Answer from the drawing. Dimensions are ordinates in mm from the lowest x, y and z of the part. A direction names the side the tool comes from. Round coordinates to 2 decimals unless told otherwise and drop trailing zeros. Loops run counter-clockwise (first coordinate to the right, second up) from the corner with the lowest first, then second, coordinate; pieces in that order, holes last. Notation, with made-up numbers: M -6.75,58.25 L 46.25,58.25 A25 cw 46.25,93.25 Z; hole C -38,-9 d8. An arc over 180 degrees is marked long. Answer as a JSON object with one key per item and string values.
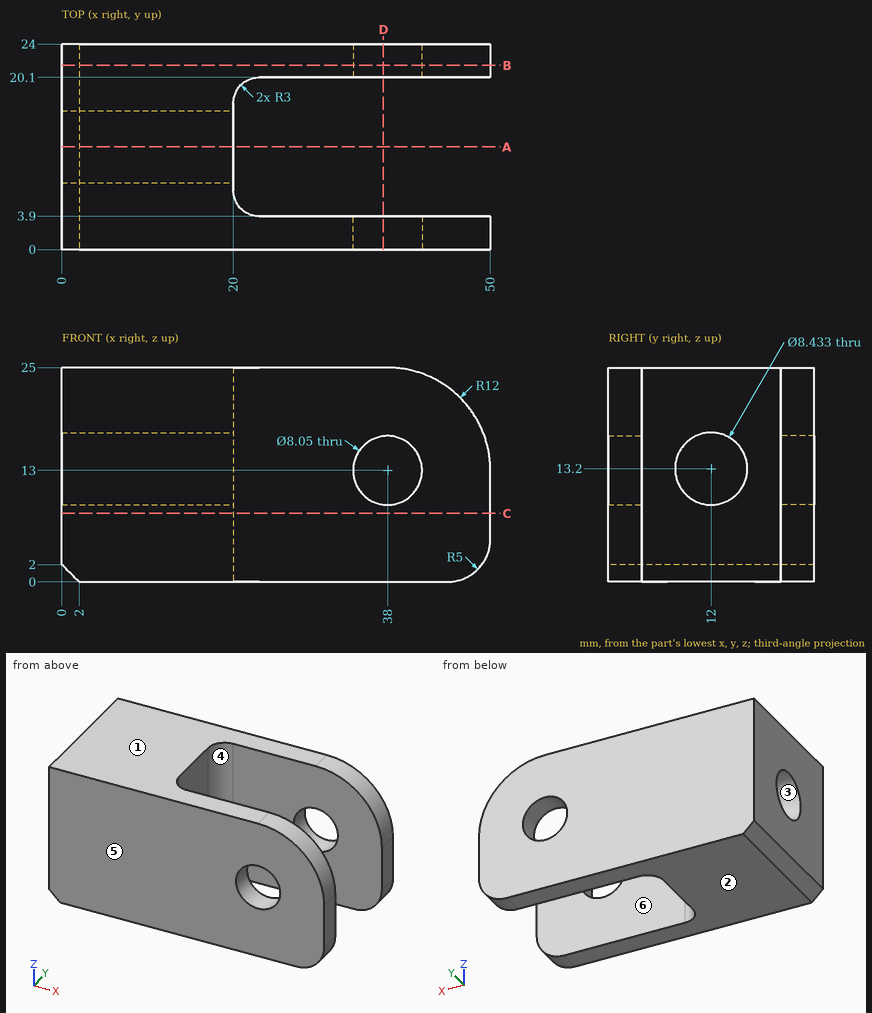
Item 1: Which of the six approach directions +Z, -Z, +X, -X, +Y, -Y give full straight-line access (tool end or side, diameter ignored) to the marked faces 5 and 6?
Values follow:
{"face 5": "+Z, -Z, +X, -X, -Y", "face 6": "+Z, -Z, +X"}
Item 2: Determine the mould class of the marked faces 1, 2, 3 and 4 for opening direction Z: released by +Z, released by -Z, zero draft, split by the parting line, or undercut.
Values follow:
{"face 1": "released by +Z", "face 2": "released by -Z", "face 3": "undercut", "face 4": "zero draft"}
Item 3: Straight lines are drawn through the part: line 1 (Y direction, x = 24, z = 16.75); line 2 (X direction, y = 2.5, z = 13.25); line 3 (Z direction, x = 13.75, y = 12). For each, find the intervals that lie inside material, in ascending order.
Values follow:
{"line 1": "0 to 3.9, 20.1 to 24", "line 2": "0 to 33.98, 42.02 to 50", "line 3": "0 to 8.98, 17.42 to 25"}
Item 4: The part is cut by section A-A (y = 12). Give the vertices of the cut face in (x, z).
Values follow:
{"outline": "M 0,2 L 2,0 L 20,0 L 20,8.98 L 0,8.98 Z; M 0,17.42 L 20,17.42 L 20,25 L 0,25 Z"}
Item 5: The part is cut by section C-C (z = 8). Give the vertices of the cut face in (x, y).
Values follow:
{"outline": "M 0,0 L 50,0 L 50,3.9 L 23,3.9 A3 cw 20,6.9 L 20,17.1 A3 cw 23,20.1 L 50,20.1 L 50,24 L 0,24 Z"}
Item 6: The part is cut by section D-D (x = 37.5). Give the vertices of the cut face in (y, z), then the cut area to 3 significant figures.
Values follow:
{"outline": "M 0,0 L 3.9,0 L 3.9,9.01 L 0,9.01 Z; M 0,16.99 L 3.9,16.99 L 3.9,25 L 0,25 Z; M 20.1,0 L 24,0 L 24,9.01 L 20.1,9.01 Z; M 20.1,16.99 L 24,16.99 L 24,25 L 20.1,25 Z", "area": "133 mm^2"}
Item 7: Flat-ended cylindrical pins translate along their axes: P1, Ø13.5, axis at y = 12, z = 13.2, coming from the -X side; P2, Ø6, axis at y = 8, z = 5.5, coming from the +X side; P3, Ø5, axis at y = 10.5, z = 9.5, coming from the +X side. Find the tip coordinate at first contact, or state that the pin passes through.
Values follow:
{"P1": "x = 0", "P2": "x = 20.68", "P3": "x = 20"}
Item 8: The part is cut by section B-B (y = 21.5). Give the vertices of the cut face in (x, z) (3 decimals).
Values follow:
{"outline": "M 0,2 L 2,0 L 45,0 A5 ccw 50,5 L 50,13 A12 ccw 38,25 L 0,25 Z; hole C 38,13 d8.05"}
